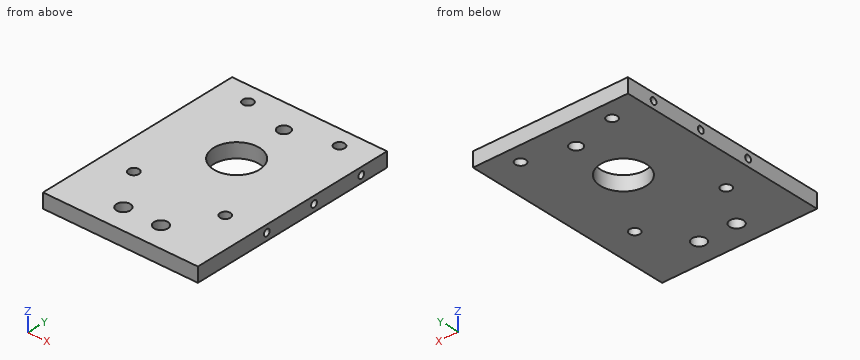
```python
from build123d import *

# Parameters (mm, degrees)
CROQUIS1_W              = 101.6
CROQUIS1_H              = 108
SALIENTE_EXTRUIR1_DEPTH = 9.525
CROQUIS2_R              = 15
CROQUIS2_R_2            = 3.4
CORTAR_EXTRUIR1_DEPTH   = 10.525
CROQUIS3_R              = 2.15
CORTAR_EXTRUIR2_DEPTH   = 15
CROQUIS4_R              = 2.15
CORTAR_EXTRUIR3_DEPTH   = 15
CROQUIS5_W              = 101.6
CROQUIS5_H              = 32
SALIENTE_EXTRUIR2_DEPTH = 9.525
CROQUIS6_R              = 4.5
CROQUIS6_R_2            = 4
CORTAR_EXTRUIR4_DEPTH   = 101.6


with BuildPart() as part:
    # Croquis1 → Saliente-Extruir1 (new body)
    with BuildSketch(Plane.XY):
        Rectangle(CROQUIS1_W, CROQUIS1_H)
    extrude(amount=SALIENTE_EXTRUIR1_DEPTH)

    # Croquis2 → Cortar-Extruir1 (cut, through all)
    with BuildSketch(Plane.XY.offset(9.525)):
        Circle(CROQUIS2_R)
        with Locations((30, -42.25)):
            Circle(CROQUIS2_R_2)
        with Locations((-30, -42.25)):
            Circle(CROQUIS2_R_2)
        with Locations((30, 42.25)):
            Circle(CROQUIS2_R_2)
        with Locations((-30, 42.25)):
            Circle(CROQUIS2_R_2)
    extrude(amount=-CORTAR_EXTRUIR1_DEPTH, mode=Mode.SUBTRACT)

    # Croquis3 → Cortar-Extruir2 (cut)
    with BuildSketch(Plane.ZY.offset(50.8)):
        with Locations((4.7625, 0)):
            Circle(CROQUIS3_R)
        with Locations((4.7625, -35)):
            Circle(CROQUIS3_R)
        with Locations((4.7625, 35)):
            Circle(CROQUIS3_R)
    extrude(amount=-CORTAR_EXTRUIR2_DEPTH, mode=Mode.SUBTRACT)

    # Croquis4 → Cortar-Extruir3 (cut)
    with BuildSketch(Plane(origin=(50.8, 0, 0), x_dir=(0, 0, -1), z_dir=(1, 0, 0))):
        with Locations((-4.7625, 0)):
            Circle(CROQUIS4_R)
        with Locations((-4.7625, -35)):
            Circle(CROQUIS4_R)
        with Locations((-4.7625, 35)):
            Circle(CROQUIS4_R)
    extrude(amount=-CORTAR_EXTRUIR3_DEPTH, mode=Mode.SUBTRACT)

    # Croquis5 → Saliente-Extruir2 (add)
    with BuildSketch(Plane.XY.offset(9.525)):
        with Locations((0, -70)):
            Rectangle(CROQUIS5_W, CROQUIS5_H)
    extrude(amount=-SALIENTE_EXTRUIR2_DEPTH)

    # Croquis6 → Cortar-Extruir4 (cut)
    with BuildSketch(Plane.XY.offset(9.525)):
        with Locations((12.329020614, -69.921350464)):
            Circle(CROQUIS6_R)
        with Locations((-12.329020614, -69.921350464)):
            Circle(CROQUIS6_R)
        with Locations((0, 35.004884714)):
            Circle(CROQUIS6_R_2)
    extrude(amount=-CORTAR_EXTRUIR4_DEPTH, mode=Mode.SUBTRACT)


solid = part.part
```
The model under review builds one solid part; all positions refer to its coordinate system, in mm. Round coordinates to 2 decimals unless told otherwise and drop trailing zeros. Order: outer loops, then holes, each group sorted by start corner. A loop starts at its lowest first (then second) coordinate and runs counter-clockwise, first axis right, second up. Notation, with made-up numbers: M 83,58 L 87,58 A15 cw 87,79 Z; hole C 51,45 d7. An arc over 180 degrees is marked long. Use a Markdown table: item, result.
1) Consider section A-A (y = -42.25). Write out the cut boundary in (x, z) (3 decimals), then the cut area to 3 significant figures.
Report:
| item | result |
|---|---|
| outline | M -50.8,0 L -33.4,0 L -33.4,9.525 L -50.8,9.525 Z; M -26.6,0 L 26.6,0 L 26.6,9.525 L -26.6,9.525 Z; M 33.4,0 L 50.8,0 L 50.8,9.525 L 33.4,9.525 Z |
| area | 838 mm^2 |
2) Consider section C-C (y = 0). Write out the cut boundary in (x, z) (1 decimal), then the cut area to 3 significant figures.
Report:
| item | result |
|---|---|
| outline | M -50.8,0 L -15,0 L -15,9.5 L -50.8,9.5 L -50.8,6.9 L -35.8,6.9 L -35.8,2.6 L -50.8,2.6 Z; M 15,0 L 50.8,0 L 50.8,2.6 L 35.8,2.6 L 35.8,6.9 L 50.8,6.9 L 50.8,9.5 L 15,9.5 Z |
| area | 553 mm^2 |
3) Wall thickness on line 1 along X through (y, z) = (-42, 2); line 2 along Y through (x, z) = (0, 4.5); line 3 along X through (y, z) = (1, 4): over which ranges is each line inside the solid? List them lowest first. Write a range as [from, to].
Report:
| item | result |
|---|---|
| line 1 | [-50.8, -33.39], [-26.61, 26.61], [33.39, 50.8] |
| line 2 | [-86, -15], [15, 31], [39, 54] |
| line 3 | [-35.8, -14.97], [14.97, 35.8] |
4) Insertion check: pin 1 (2.5 mm diameter, centred on y = -35, z = 4.76, fed in from +X); pin 2 (5.5 mm diameter, centred on x = 30, y = -42.25, fed in from +Z) (3 decimals); pin 3 (2 mm diameter, centred on y = -1, z = 4.5, fed in from -X). Each pin has a flat end and moves straight along its axis. Give the tip position at first contact, or say it passes through.
Report:
| item | result |
|---|---|
| pin 1 | x = 35.8 |
| pin 2 | through |
| pin 3 | x = -35.8 |
5) Consider section D-D (z = 4.5). Give the number of separate pieces and of enclosed holes in the cut face, then the cut area to 3 significant figures.
Report:
| item | result |
|---|---|
| separate pieces | 1 |
| enclosed holes | 8 |
| area | 12,800 mm^2 |
6) Consider section B-B (x = 30). Write out the cut boundary in (y, z) (3 decimals), then the cut area to 3 significant figures.
Report:
| item | result |
|---|---|
| outline | M -86,0 L -45.65,0 L -45.65,9.525 L -86,9.525 Z; M -38.85,0 L 38.85,0 L 38.85,9.525 L -38.85,9.525 Z; M 45.65,0 L 54,0 L 54,9.525 L 45.65,9.525 Z |
| area | 1,200 mm^2 |
